For this review, use the dimensioned drawing (mm, ordinates from the lowest corner) and the shaded views. A direction names the side the tool comes from. Give positions to 0.01 mm unless a question says otherwise; leave off trailing zeros. Loops run counter-clockwise (first coordinate to the right, second up) from the corner with the lowest first, then second, coordinate; pieces in that order, holes last. Notation, with made-up numbers: (26.25, 84) -> (45.25, 84) arc R36 cw to (45.25, 123) -> close; hole circle Ø5 at (72.5, 13). An arc over 180 degrees is marked (long way). Use a Markdown table: item, result. Add a question column.
1. Draft analysis for pull direction Y (two halves, no side actions). For the marked faces 4, 5 and 6, state which applies: pulls with the +Y half, pulls with the -Y half, needs draft (parallel to the pull), parting line crosses it, or undercut.
2. Add section A-A (z = 15). State the section outline as (x, y) points (1 decimal), and give its area (3 significant figures).
3. Add section B-B (z = 71). State the section outline as (x, y) points (1 decimal), and give its area (3 significant figures).
4. For pin 1 Ø3 at (x, y) = (51.5, 66) entering from -Z; pin 2 Ø5 at (x, z) = (68, 53.5) entering from +Y; pin 3 Ø1 at (y, z) = (22.5, 68) entering from +X; pin 4 Ø8 at (x, y) = (39, 47) entering from -Z, all flat-tipped, find the tip position at first contact; note any pin that passes through.
5. For the marked faces 1, 2 and 3, list the 3-axis set-ups (+Z, -Z, +X, -X, +Y, -Y) from which the entire face can be reached by the end or side of a thin tool; tool diameter is ignored.
6. To check wall thickness, follow line 1 (X direction, y = 43, z = 59); line 2 (Z direction, x = 33.5, y = 58); line 3 (Y direction, x = 40, z = 12). State the ranges of each line that lie inside material, in increasing order.
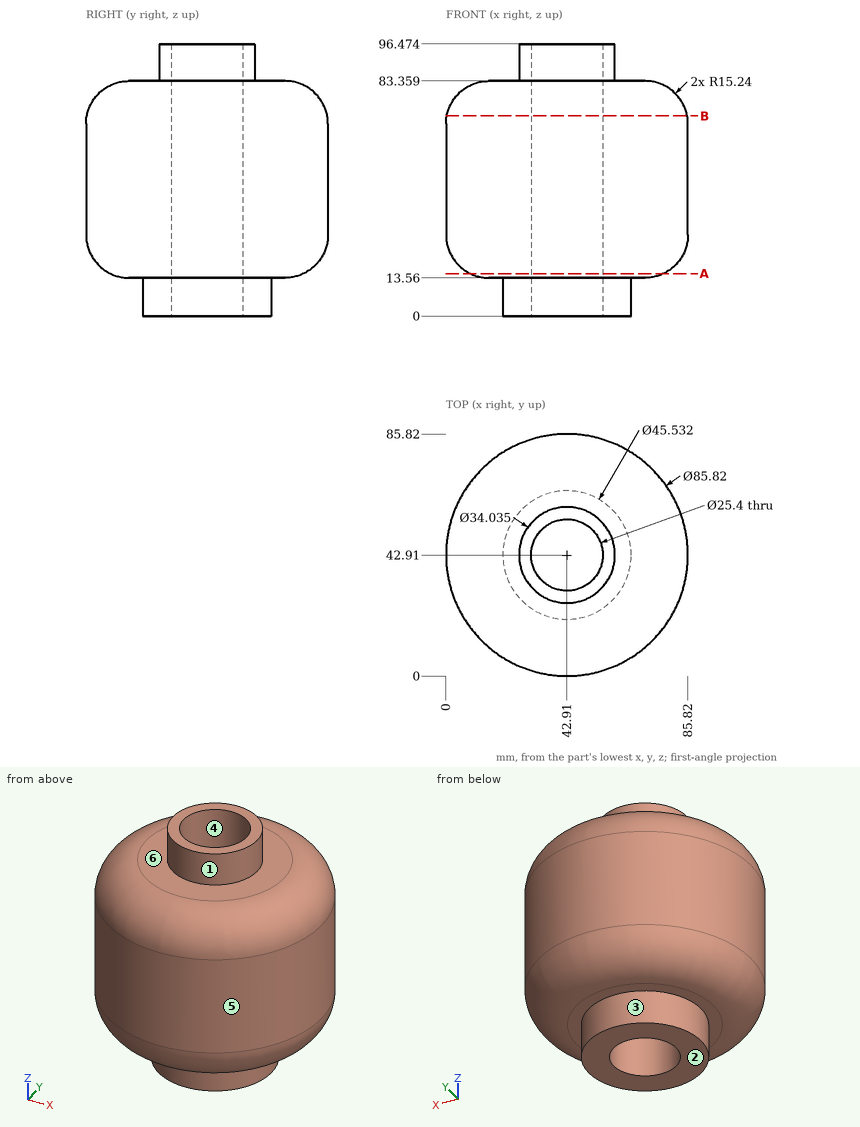
Taken from the geometry:
| question | item | result |
|---|---|---|
| 1 | face 4 | undercut |
| 1 | face 5 | parting line crosses it |
| 1 | face 6 | needs draft |
| 2 | outline | circle Ø68.3 at (42.9, 42.9); hole circle Ø25.4 at (42.9, 42.9) |
| 2 | area | 3,150 mm^2 |
| 3 | outline | circle Ø85.3 at (42.9, 42.9); hole circle Ø25.4 at (42.9, 42.9) |
| 3 | area | 5,200 mm^2 |
| 4 | pin 1 | stops at z = 13.56 |
| 4 | pin 2 | stops at y = 79.39 |
| 4 | pin 3 | stops at x = 80.92 |
| 4 | pin 4 | passes through |
| 5 | face 1 | +Z |
| 5 | face 2 | -Z, +X, -X, +Y, -Y |
| 5 | face 3 | -Z |
| 6 | line 1 | x = 0 to 30.21, 55.61 to 85.82 |
| 6 | line 2 | z = 0 to 83.36 |
| 6 | line 3 | y = 20.33 to 30.55, 55.27 to 65.49 |
